Autodesk Inventor part; units mm, degrees
ref_plane "YZ Plane" through (0, 0, 0) normal (1, 0, 0) x (0, 1, 0)
ref_plane "XZ Plane" through (0, 0, 0) normal (0, 1, 0) x (-1, 0, 0)
ref_plane "XY Plane" through (0, 0, 0) normal (0, 0, 1) x (1, 0, 0)
sketch "Sketch1" plane through (0, 0, 0) normal (0, 0, 1) x (1, 0, 0)
  line L0 (0, 0) -> (15, 0)
  line L1 (16, 1) -> (16, 45)
  line L2 (15, 46) -> (-15, 46)
  line L3 (-16, 45) -> (-16, 1)
  line L4 (-15, 0) -> (16, 0)
  arc A0 (-15, 46) -> (-16, 45) centre (-15, 45) ccw
  arc A1 (16, 45) -> (15, 46) centre (15, 45) ccw
  arc A2 (15, 0) -> (16, 1) centre (15, 1) ccw
  arc A3 (-16, 1) -> (-15, 0) centre (-15, 1) ccw
  point P0 (16, 46)
  point P1 (-16, 46)
  dimension "d0" = 16
  dimension "d1" = 46
  dimension "d2" = 32
  dimension "d3" = 1
extrude "Extrusion1" add sketch "Sketch1" along normal blind 22.5
sketch "Sketch2" plane through (0, 0, 0) normal (0, 0, -1) x (-1, 0, 0)
  line L0 (0, 0) -> (-10, 0)
  line L1 (15, 0) -> (-15, 0)
  line L2 (-10, 0) -> (-10, 7)
  line L3 (-10, 7) -> (-10, 40)
  circle A0 centre (-10, 7) radius 3.7
  circle A1 centre (-10, 40) radius 3.7
  line L4 (-10, 40) -> (8, 40)
  line L5 (-10, 7) -> (8, 7)
  circle A2 centre (8, 7) radius 3.7
  circle A3 centre (8, 40) radius 3.7
  line L6 (-15, 46) -> (15, 46)
  line L7 (0, 46) -> (0, 31)
  circle A4 centre (0, 31) radius 6
  dimension "d6" = 10
  dimension "d7" = 7
  dimension "d8" = 33
  dimension "d9" = 7.4
  dimension "d10" = 7.4
  dimension "d11" = 18
  dimension "d12" = 18
  dimension "d13" = 7.4
  dimension "d14" = 7.4
  dimension "d23" = 15
  dimension "d24" = 12
extrude "Extrusion2" add sketch "Sketch2" along normal blind 2
sketch "Sketch3" plane through (10, 7, -2) normal (0, 0, -1) x (-1, 0, 0)
  circle A0 centre (0, 0) radius 3.7
  circle A1 centre (0, 0) radius 1.5
  circle A2 centre (0, 33) radius 3.7
  circle A3 centre (0, 33) radius 1.5
  circle A4 centre (18, 33) radius 3.7
  circle A5 centre (18, 33) radius 1.5
  circle A6 centre (18, 0) radius 3.7
  circle A7 centre (18, 0) radius 1.5
  point P0 (10, -7)
  dimension "d17" = 3
  dimension "d18" = 3
  dimension "d19" = 3
  dimension "d20" = 3
extrude "Extrusion3" cut sketch "Sketch3" against normal blind 3 contours A1 | A3 | A5 | A7
sketch "Sketch4" plane through (0, 31, -2) normal (0, 0, -1) x (-1, 0, 0)
  circle A0 centre (0, 0) radius 6
  circle A1 centre (0, 0) radius 3
  point P0 (0, -31)
  dimension "d25" = 6
extrude "Extrusion4" add sketch "Sketch4" along normal blind 18.5 contours A1
sketch "Sketch5" plane through (0, 31, -20.5) normal (0, 0, -1) x (-1, 0, 0)
  circle A0 centre (0, 0) radius 3
  line L0 (0, 3) -> (0, -2.4)
  line L1 (0, -2.4) -> (-1.8, -2.4)
  line L2 (0, -2.4) -> (1.8, -2.4)
  point P0 (0, -31)
  dimension "d28" = 5.4
extrude "Extrusion5" cut sketch "Sketch5" against normal blind 10 contours A0 L1 L2
sketch "Sketch6" plane through (-15, 0, 0) normal (0, -1, 0) x (1, 0, 0)
  circle A0 centre (11.8, 13.2) radius 12.2
  line L0 (-1, 0) -> (-1, 22.5)
  line L1 (0, 0) -> (30, 0)
  point P0 (15, 0)
  dimension "d31" = 24.4
  dimension "d40" = 13.2
  dimension "d41" = 12.8
extrude "Extrusion6" add sketch "Sketch6" along normal blind 30.8
sketch "Sketch7" plane through (-3.2, -30.8, 13.2) normal (0, -1, 0) x (1, 0, 0)
  line L0 (0, 0) -> (10, 0)
  line L1 (10, 0) -> (10, -2)
  line L2 (10, -2) -> (10, 2)
  line L3 (10, 2) -> (9, 2)
  line L4 (9, 2) -> (9, -2)
  line L5 (9, -2) -> (10, -2)
  line L6 (0, 0) -> (0, -2)
  line L7 (0, 0) -> (-10, 0)
  line L8 (-10, 0) -> (-10, -2)
  line L9 (-10, -2) -> (-10, 2)
  line L10 (-10, 2) -> (-9, 2)
  line L11 (-9, 2) -> (-9, -2)
  line L12 (-9, -2) -> (-10, -2)
  point P0 (3.2, -13.2)
  dimension "d34" = 10
  dimension "d35" = 2
  dimension "d36" = 4
  dimension "d37" = 1
extrude "Extrusion7" add sketch "Sketch7" along normal blind 4.2
equation "\"d0\" = 0.5 * d2"
properties part number "motor_dc_12v_90d"
Read the model definition and answer for the solid it produces. Units are mm, in the model's axes. A direction names the side the tool comes from. Coordinates: 2 decimals unless noted, no trailing zeros. Write each loop counter-clockwise with the first axis right and the second up, starting at its lowest first coordinate (ties: lowest second). Pieces come first, ordered by that corner, then holes. Notation, with made-up numbers: (16.25, -34) - (41.25, -34) arc R18 cw to (41.25, -26) - close; hole circle Ø10 at (39.25, 85). An arc over 180 degrees is marked (long way). Answer as a JSON object with one key per item and string values. Group by question number.
1. The mould has two halves that part along Y. Classify faces 1 (the flat face through (-8, 40, 1)), 2 (the flat face through (-16, 23, 11)), 3 (the flat face through (0, 46, 11)): +Y half, -Y half, draft (parallel to the pull), parting line (faces both ways), or undercut.
2. A cutting plane is placed at B-B (x = 10). Determine the outline of the cut face in (y, z).
3. Each of these flat-tipped pins is pushed along its axis until it touches: P1, Ø8, axis at x = -12, y = -1.5, coming from the -Z side; P2, Ø5, axis at x = 10, y = 7, coming from the -Z side; P3, Ø6, axis at x = 5, y = 11, coming from the +Z side; P4, Ø0.5, axis at x = 0, y = 28.5, coming from the -Z side. Where does it stop, or does it pass through?
4. Consider L1, parallel to Y at x = 10, z = 0.05; L2, parallel to Y at x = -8, z = -0.3; L3, parallel to Y at x = -5, z = 11.5. Determine where each line is inside the solid, lowest interval first. Write a range as [from, to].
5. A cutting plane is placed at A-A (y = 31). Determine the outline of the cut face in (x, z), plus the area to 3 significant figures.
6. Which of the six approach directions +Z, -Z, +X, -X, +Y, -Y give full straight-line access (tool end or side, diameter ignored) to faces 4 (the flat face through (-13.2, -33, 13)), 5 (the flat face through (6.8, -33, 13)), 6 (the flat face through (0, 23, 22.5)), 7 (the flat face through (3, 30, -2))?
7. A cutting plane is placed at C-C (z = 13.2). Determine the outline of the cut face in (x, y).
8. A cutting plane is placed at D-D (y = 13.5). Determine the outline of the cut face in (x, z), plus the area to 3 significant figures.
Worked out:
{
 "1": {"face 1": "undercut", "face 2": "draft", "face 3": "+Y half"},
 "2": {"outline": "(0, 0) - (3.3, 0) - (3.3, -2) - (5.5, -2) - (5.5, 1) - (8.5, 1) - (8.5, -2) - (10.7, -2) - (10.7, 0) - (36.3, 0) - (36.3, -2) - (38.5, -2) - (38.5, 1) - (41.5, 1) - (41.5, -2) - (43.7, -2) - (43.7, 0) - (46, 0) - (46, 22.5) - (0, 22.5) - close"},
 "3": {"P1": "stops at z = 0", "P2": "stops at z = -2", "P3": "stops at z = 22.5", "P4": "stops at z = -20.5"},
 "4": {"L1": "y = [0, 5.5], [8.5, 38.5], [41.5, 46]", "L2": "y = [3.3, 5.5], [8.5, 10.7], [36.3, 38.5], [41.5, 43.7]", "L3": "y = [-30.8, 46]"},
 "5": {"outline": "(-16, 0) - (-6, 0) - (-6, -2) - (-3, -2) - (-3, -20.5) - (3, -20.5) - (3, -2) - (6, -2) - (6, 0) - (16, 0) - (16, 22.5) - (-16, 22.5) - close", "area": "855 mm²"},
 "6": {"face 4": "+Z, -Z, -X, -Y", "face 5": "+Z, -Z, +X, -Y", "face 6": "+Z, +X, -X, +Y", "face 7": "-Z"},
 "7": {"outline": "(-16, 1) arc R1 ccw to (-15, 0) - (-15.4, 0) - (-15.4, -30.8) - (-13.2, -30.8) - (-13.2, -35) - (-12.2, -35) - (-12.2, -30.8) - (5.8, -30.8) - (5.8, -35) - (6.8, -35) - (6.8, -30.8) - (9, -30.8) - (9, 0) - (15, 0) arc R1 ccw to (16, 1) - (16, 45) arc R1 ccw to (15, 46) - (-15, 46) arc R1 ccw to (-16, 45) - close"},
 "8": {"outline": "(-16, 0) - (16, 0) - (16, 22.5) - (-16, 22.5) - close", "area": "720 mm²"}
}
